Design review of the part built by this model. Coordinates are the model's own, in mm. A direction names the side the tool comes from. Give positions to 0.01 mm unless a question says otherwise; leave off trailing zeros. Write each loop counter-clockwise with the first axis right and the second up, starting at its lowest first coordinate (ties: lowest second). Pieces come first, ordered by that corner, then holes. Notation, with made-up numbers: (73.5, -30) -> (128.5, -30) arc R27 ccw to (128.5, 1) -> close; hole circle Ø10 at (-9.75, 87). An arc over 180 degrees is marked (long way). Answer as a JSON object with one key per item and string values.
```python
from build123d import *

# Parameters (mm, degrees)
BOSS_EXTRUDE1_DEPTH = 3
SKETCH1_3_W         = 3
SKETCH1_3_H         = 45.75
SKETCH1_3_H_2       = 39.75
BOSS_EXTRUDE2_DEPTH = 9
SKETCH1_4_W         = 3
SKETCH1_4_H         = 45.75
BOSS_EXTRUDE3_DEPTH = 6
CUT_EXTRUDE1_REACH  = 47.678
SKETCH3_R           = 1.35
SKETCH1_5_W         = 3
SKETCH1_5_H         = 3
BOSS_EXTRUDE4_DEPTH = 20
BOSS_EXTRUDE5_DEPTH = 3
SKETCH5_R           = 2.25
SKETCH5_R_2         = 1.1
CUT_EXTRUDE2_DEPTH  = 3
SKETCH6_R           = 1.6
CUT_EXTRUDE3_DEPTH  = 3
CIRPATTERN1_COUNT   = 4
CUT_EXTRUDE4_REACH  = 93.224


with BuildPart() as part:
    # Sketch1 → Boss-Extrude1 (new body)
    with BuildSketch(Plane(origin=(0, 0, 0), x_dir=(1, 0, 0), z_dir=(0, 1, 0))):
        Polygon((16.25, 22.875), (-16.25, 22.875), (-16.25, -22.875), (16.25, -22.875), (16.25, -19.875), (16.25, 19.875), align=None)
    extrude(amount=-BOSS_EXTRUDE1_DEPTH)

    # Sketch1<3> → Boss-Extrude2 (add)
    with BuildSketch(Plane(origin=(0, 0, 0), x_dir=(1, 0, 0), z_dir=(0, 1, 0))):
        with Locations((-17.75, 0)):
            Rectangle(SKETCH1_3_W, SKETCH1_3_H)
        with Locations((17.75, 0)):
            Rectangle(SKETCH1_3_W, SKETCH1_3_H_2)
    extrude(amount=-BOSS_EXTRUDE2_DEPTH)

    # Sketch1<4> → Boss-Extrude3 (add)
    with BuildSketch(Plane(origin=(0, 0, 0), x_dir=(1, 0, 0), z_dir=(0, 1, 0))):
        with Locations((-17.75, 0)):
            Rectangle(SKETCH1_4_W, SKETCH1_4_H)
    extrude(amount=-BOSS_EXTRUDE3_DEPTH)

    # Cut-Extrude1: up to this face of the body (flat: up to its plane)
    cut_extrude1_end = Plane(part.part.faces().sort_by_distance((19.25, -4.5, 0))[0])
    # Sketch3 → Cut-Extrude1 (cut, up to the picked face)
    with BuildSketch(Plane.ZY.offset(19.25), mode=Mode.PRIVATE) as cut_extrude1_sk1:
        with Locations((-8, -5.5)):
            Circle(SKETCH3_R)
    cut_extrude1_tool1 = split(extrude(cut_extrude1_sk1.sketch, amount=-CUT_EXTRUDE1_REACH, mode=Mode.PRIVATE), bisect_by=cut_extrude1_end, keep=Keep.BOTH, mode=Mode.PRIVATE)
    cut_extrude1 = cut_extrude1_tool1.solids().sort_by(Axis((-19.25, -5.5, -8), (1, 0, 0)))[0]
    add(cut_extrude1, mode=Mode.SUBTRACT)

    # Mirror1: Cut-Extrude1 across plane
    add(cut_extrude1.mirror(Plane.XY), mode=Mode.SUBTRACT)

    # Sketch1<5> → Boss-Extrude4 (add)
    with BuildSketch(Plane(origin=(0, 0, 0), x_dir=(1, 0, 0), z_dir=(0, 1, 0))):
        with Locations((17.75, 21.375)):
            Rectangle(SKETCH1_5_W, SKETCH1_5_H)
        with Locations((17.75, -21.375)):
            Rectangle(SKETCH1_5_W, SKETCH1_5_H)
    extrude(amount=-BOSS_EXTRUDE4_DEPTH)

    # Sketch4 → Boss-Extrude5 (add)
    with BuildSketch(Plane.XY.offset(22.875)):
        with BuildLine():
            Line((19.25, -4), (53.343559989, -38.311496139))
            ThreePointArc((53.343559989, -38.311496139), (52.66855868, -53.028253026), (38.062810036, -51.101943964))
            Line((38.062810036, -51.101943964), (16.25, -20))
            Line((16.25, -20), (19.25, -4))
        make_face()
    boss_extrude5 = extrude(amount=-BOSS_EXTRUDE5_DEPTH)

    # Mirror2: Boss-Extrude5 across plane
    add(boss_extrude5.mirror(Plane.XY))

    # Sketch5 → Cut-Extrude2 (cut)
    with BuildSketch(Plane.XY.offset(22.875)):
        with Locations((46.25, -45.36)):
            Circle(SKETCH5_R)
        with Locations((51.906854249, -39.703145751)):
            Circle(SKETCH5_R_2)
    cut_extrude2 = extrude(amount=-CUT_EXTRUDE2_DEPTH, mode=Mode.SUBTRACT)

    # Sketch6 → Cut-Extrude3 (cut)
    with BuildSketch(Plane(origin=(0, 0, -22.875), x_dir=(-1, 0, 0), z_dir=(0, 0, -1))):
        with Locations((-46.25, -45.36)):
            Circle(SKETCH6_R)
    extrude(amount=-CUT_EXTRUDE3_DEPTH, mode=Mode.SUBTRACT)

    # CirPattern1: Cut-Extrude2 ×4 about axis
    cirpattern1_axis = Axis((46.25, -45.36, 0), (0, 0, 1))
    for i in range(1, CIRPATTERN1_COUNT):
        add(cut_extrude2.rotate(cirpattern1_axis, i * 360 / CIRPATTERN1_COUNT), mode=Mode.SUBTRACT)

    # Cut-Extrude4: up to this face of the body (flat: up to its plane)
    cut_extrude4_end = Plane(part.part.faces().sort_by_distance((30.534092, -28.25383722, -22.875))[0])
    # Sketch7 → Cut-Extrude4 (cut, up to the picked face)
    with BuildSketch(Plane.XY.offset(22.875), mode=Mode.PRIVATE) as cut_extrude4_sk1:
        with BuildLine():
            Line((27.924933355, -12.730386103), (30.7443349, -15.567810098))
            ThreePointArc((30.7443349, -15.567810098), (27.915922129, -15.558798873), (27.924933355, -12.730386103))
        make_face()
    cut_extrude4_tool1 = split(extrude(cut_extrude4_sk1.sketch, amount=-CUT_EXTRUDE4_REACH, mode=Mode.PRIVATE), bisect_by=cut_extrude4_end, keep=Keep.BOTH, mode=Mode.PRIVATE)
    add(cut_extrude4_tool1.solids().sort_by(Axis((28.732514, -14.747394, 22.875), (0, 0, -1)))[0], mode=Mode.SUBTRACT)


solid = part.part
```
(1) We need section C-C, the plane x = 46.25. State the section outline as (y, z) points (3 decimals), then the cut area to 3 significant figures.
Here are the results:
{"outline": "(-55.36, -22.875) -> (-46.96, -22.875) -> (-46.96, -19.875) -> (-55.36, -19.875) -> close; (-55.36, 19.875) -> (-47.61, 19.875) -> (-47.61, 22.875) -> (-55.36, 22.875) -> close; (-43.76, -22.875) -> (-31.173, -22.875) -> (-31.173, -19.875) -> (-43.76, -19.875) -> close; (-43.11, 19.875) -> (-31.173, 19.875) -> (-31.173, 22.875) -> (-43.11, 22.875) -> close", "area": "122 mm²"}
(2) For faces 1 (the flat face through (18, -9, 0)), 2 (the flat face through (16.25, -8, 0)), 3 (the flat face through (-18, -9, 0)), 4 (the cylindrical face through (41.47, -50.35, 21.4)), 5 (the cylindrical face through (-17.771, -5.094, 6.712)), list the 3-axis set-ups (+Z, -Z, +X, -X, +Y, -Y) from which the entire face can be reached by the end or side of a thin tool; tool diameter is ignored.
Here are the results:
{"face 1": "+X, -X, -Y", "face 2": "+Z, -Z, -Y", "face 3": "+Z, -Z, -X, -Y", "face 4": "+Z", "face 5": "+X, -X"}
(3) We need section B-B, the plane y = -45.36. State the section outline as (x, z) points (3 decimals), then the cut area to 3 significant figures.
Here are the results:
{"outline": "(34.036, -22.875) -> (44.65, -22.875) -> (44.65, -19.875) -> (34.036, -19.875) -> close; (34.036, 19.875) -> (44, 19.875) -> (44, 22.875) -> (34.036, 22.875) -> close; (47.85, -22.875) -> (56.25, -22.875) -> (56.25, -19.875) -> (47.85, -19.875) -> close; (48.5, 19.875) -> (56.25, 19.875) -> (56.25, 22.875) -> (48.5, 22.875) -> close", "area": "110 mm²"}
(4) We need section D-D, the plane y = -22. State the section outline as (x, z) points (3 decimals).
Here are the results:
{"outline": "(17.653, -22.875) -> (37.136, -22.875) -> (37.136, -19.875) -> (17.653, -19.875) -> close; (17.653, 19.875) -> (37.136, 19.875) -> (37.136, 22.875) -> (17.653, 22.875) -> close"}
(5) The part is to be moulded in two halves that separate along Y. For faces 6 (the cylindrical face through (50.81, -39.65, 21.4)), 7 (the cylindrical face through (52.84, -52.88, 21.4)), 8 (the flat face through (30, -28, -22.875)), say which applies: +Y half, -Y half, draft (parallel to the pull), parting line (faces both ways), or undercut.
Here are the results:
{"face 6": "undercut", "face 7": "parting line", "face 8": "draft"}
(6) For line 1 along Y through (x, z) = (17.2, 8); line 2 along Z through (x, y) = (49, -37) (3 decimals); line 3 along Y through (x, z) = (16, 17), list the stretches that pass through material, from the lowest coordinate up.
Here are the results:
{"line 1": "y = -9 to -6.85, -4.15 to 0", "line 2": "z = -22.875 to -19.875, 19.875 to 22.875", "line 3": "y = -3 to 0"}
(7) We need section A-A, the plane z = 8. State the section outline as (x, y) points.
Here are the results:
{"outline": "(-19.25, -9) -> (-16.25, -9) -> (-16.25, -6.85) -> (-19.25, -6.85) -> close; (-19.25, -4.15) -> (-16.25, -4.15) -> (-16.25, -3) -> (16.25, -3) -> (16.25, -4.15) -> (19.25, -4.15) -> (19.25, 0) -> (-19.25, 0) -> close; (16.25, -9) -> (19.25, -9) -> (19.25, -6.85) -> (16.25, -6.85) -> close"}
(8) Clearance check with flat-ended pins moving along their axes: pin 1 (3 mm diameter, centred on y = -5.5, z = 6, fed in from +X); pin 2 (10 mm diameter, centred on x = 3.5, z = -4.5, fed in from -Y); pin 3 (8 mm diameter, centred on y = -49, z = -14, fed in from +X); pin 4 (2.5 mm diameter, centred on x = 17.5, z = -3, fed in from -Y). State where each tip first meets the part, or that it passes through.
Here are the results:
{"pin 1": "stops at x = 19.25", "pin 2": "stops at y = -3", "pin 3": "passes through", "pin 4": "stops at y = -9"}
